from build123d import *

# Parameters (mm, degrees)
F1_DEPTH = 15.24
F2_DEPTH = 12.7
F3_DEPTH = 15.24
F5_DEPTH = 101.6


# Not quite as in the source:
# - a feature names something its author has since deleted; it is built from what else it names


with BuildPart() as f1:
    # F0 (on Right) → F1 (new body)
    with BuildSketch(Plane.YZ):
        with BuildLine():
            ThreePointArc((37.1756509936, -4.7328671039), (19.2151387515, 2.7066206539), (11.7756509936, 20.6671328961))
            Line((11.7756509936, 20.6671328961), (-77.1243490064, 20.6671328961))
            Line((-77.1243490064, 20.6671328961), (-89.8243490064, -4.7328671039))
            Line((-89.8243490064, -4.7328671039), (37.1756509936, -4.7328671039))
        make_face()
        with BuildLine():
            Line((-77.1243490064, 20.6671328961), (11.7756509936, 20.6671328961))
            ThreePointArc((11.7756509936, 20.6671328961), (19.2151387515, 38.6276451382), (37.1756509936, 46.0671328961))
            Line((37.1756509936, 46.0671328961), (-64.4243490064, 46.0671328961))
            Line((-64.4243490064, 46.0671328961), (-77.1243490064, 20.6671328961))
        make_face()
    extrude(amount=F1_DEPTH)

    # F0 (on Right) → F2 (join)
    with BuildSketch(Plane.YZ):
        with BuildLine():
            Line((11.7756509936, 20.6671328961), (62.5756509936, 20.6671328961))
            ThreePointArc((62.5756509936, 20.6671328961), (55.1361632357, 38.6276451382), (37.1756509936, 46.0671328961))
            ThreePointArc((37.1756509936, 46.0671328961), (19.2151387515, 38.6276451382), (11.7756509936, 20.6671328961))
        make_face()
        with BuildLine():
            ThreePointArc((37.1756509936, -4.7328671039), (55.1361632357, 2.7066206539), (62.5756509936, 20.6671328961))
            Line((62.5756509936, 20.6671328961), (11.7756509936, 20.6671328961))
            ThreePointArc((11.7756509936, 20.6671328961), (19.2151387515, 2.7066206539), (37.1756509936, -4.7328671039))
        make_face()
    extrude(amount=F2_DEPTH)

    # F3 (add): a face of the model
    f3_faces = [f1.faces().sort_by_distance(p)[0] for p in [
        (7.62, -13.6243490064, 46.0671328961),
    ]]
    extrude(f3_faces, amount=F3_DEPTH)

    # F4 (on face) → F5 (cut)
    with BuildSketch(Plane.XZ.offset(64.4243490064)):
        Polygon((15.24, 61.3071328961), (0, 61.3071328961), (15.24, 46.0671328961), align=None)
    extrude(amount=-F5_DEPTH, mode=Mode.SUBTRACT)


solid = f1.part
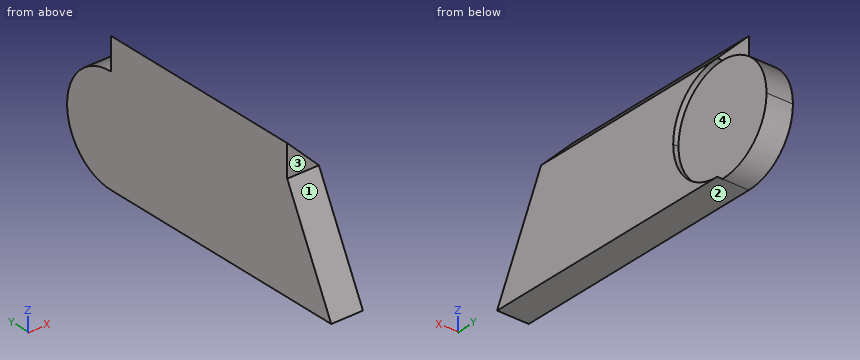
Could you check a few things on this model? Use its own coordinates, in mm. Face numbers are marked on the shaded views. Give positions to 0.01 mm unless a question says otherwise; leave off trailing zeros. Loops run counter-clockwise (first coordinate to the right, second up) from the corner with the lowest first, then second, coordinate; pieces in that order, holes last. Notation, with made-up numbers: M 47.25,-14.75 L 101.25,-14.75 A23 cw 101.25,-0.75 Z; hole C -19.75,50.5 d9. An arc over 180 degrees is marked long. Answer as a JSON object with one key per item and string values.
Q1. Suppose I cut it at A-A, the plane x = 6.75. List the corners of the cut face in (y, z) for me.
Values found:
{"outline": "M -89.82,-4.73 L 37.18,-4.73 A25.4 ccw 37.18,46.07 L 37.18,54.56 L -64.42,54.56 L -64.42,46.07 Z"}
Q2. Suppose I cut it at D-D, the plane z = 0. List the corners of the cut face in (x, y) for me, plus the area to 3 significant figures.
Values found:
{"outline": "M 0,-87.46 L 15.24,-87.46 L 15.24,22.41 L 12.7,22.41 L 12.7,51.94 L 0,51.94 Z", "area": "2,050 mm²"}
Q3. If we mould it in two halves opening along Z, with no side actions, what happens to the marked faces 1, 2, 3 and 4? For each: pulls with the +Z half, pulls with the -Z half, needs draft (parallel to the pull), parting line crosses it, or undercut.
Values found:
{"face 1": "pulls with the +Z half", "face 2": "pulls with the -Z half", "face 3": "needs draft", "face 4": "undercut"}
Q4. Suppose I cut it at C-C, the plane y = -10.5. List the corners of the cut face in (x, z) for me, plus the area to 3 significant figures.
Values found:
{"outline": "M 0,-4.73 L 15.24,-4.73 L 15.24,46.07 L 0,61.31 Z", "area": "890 mm²"}
Q5. If I drill on probe 1 along Z at (x, y) = (13.5, 28); probe 2 along Y at (x, z) = (3.5, 51); probe 3 along X at (y, z) = (26.5, 40), over which ranges is the centre line in solid material (lowest first)? Write a range as [from, to].
Values found:
{"probe 1": "z = [-4.73, -3.02], [44.35, 47.81]", "probe 2": "y = [-64.42, 37.18]", "probe 3": "x = [0, 12.7]"}
Q6. For P1, Ø2, axis at x = 6, z = 38.5, coming from the +Y side; P2, Ø3, axis at y = 17.5, z = 9, coming from the +X side, each with a flat end and sliding along its axis, tell me the tip position at first contact or that it passes through.
Values found:
{"P1": "stops at y = 56.2", "P2": "stops at x = 12.7"}
Q7. Suppose I cut it at B-B, the plane z = 26. List the corners of the cut face in (x, y) for me, plus the area to 3 significant figures.
Values found:
{"outline": "M 0,-74.46 L 15.24,-74.46 L 15.24,12.34 L 12.7,12.34 L 12.7,62.01 L 0,62.01 Z", "area": "1,950 mm²"}
